Model file for the job. Use its own axes, mm. Face numbers are marked on the shaded views. A direction names the side the tool comes from. Coordinates: 2 decimals unless noted, no trailing zeros. Order: outer loops, then holes, each group sorted by start corner. A loop starts at its lowest first (then second) coordinate and runs counter-clockwise, first axis right, second up.
from build123d import *

# Parameters (mm, degrees)
F1_DEPTH = 31.75
F2_SIZE  = 12
F4_DEPTH = 25.4
F5_R     = 3.175
F6_DEPTH = 25.4
F7_SIZE  = 5.08
F8_R     = 4.200525
F9_DEPTH = 3.175
F10_SIZE = 5.08


with BuildPart() as f1:
    # F0 (on Right) → F1 (new body, symmetric)
    with BuildSketch(Plane.YZ):
        Polygon((-72.2, 15.875), (-72.2, 0), (4, 0), (4, 76.2), (0, 76.2), (0, 6.35), (-66.2, 6.35), (-66.2, 15.875), align=None)
    extrude(amount=F1_DEPTH, both=True)

    # F2
    f2_edges = [f1.edges().sort_by_distance(p)[0] for p in [
        (0, 0, 6.35),
    ]]
    chamfer(f2_edges, length=F2_SIZE)

    # F3 (on Top) → F4 (cut)
    with BuildSketch(Plane.XY):
        with BuildLine():
            Line((-19.05, -21.518925), (-19.05, -72.2))
            Line((-19.05, -72.2), (19.05, -72.2))
            Line((19.05, -72.2), (19.05, -21.518925))
            ThreePointArc((19.05, -21.518925), (0, -8.7), (-19.05, -21.518925))
        make_face()
    extrude(amount=F4_DEPTH, mode=Mode.SUBTRACT)

    # F5 (on face) → F6 (cut)
    with BuildSketch(Plane.XZ):
        with Locations((-15.875, 67.945)):
            Circle(F5_R)
        with Locations((15.875, 67.945)):
            Circle(F5_R)
        with Locations((-15.875, 36.195)):
            Circle(F5_R)
        with Locations((15.875, 36.195)):
            Circle(F5_R)
    extrude(amount=-F6_DEPTH, mode=Mode.SUBTRACT)

    # F7
    f7_edges = [f1.edges().sort_by_distance(p)[0] for p in [
        (-25.4, -66.2, 6.35),
        (25.4, -66.2, 6.35),
    ]]
    chamfer(f7_edges, length=F7_SIZE)

    # F8 (on face) → F9 (cut)
    with BuildSketch(Plane.XZ):
        with Locations((0, 38.1)):
            Circle(F8_R)
    extrude(amount=-F9_DEPTH, mode=Mode.SUBTRACT)

    # F10
    f10_edges = [f1.edges().sort_by_distance(p)[0] for p in [
        (31.75, 2, 76.2),
        (-31.75, 2, 76.2),
        (0, 4, 0),
    ]]
    chamfer(f10_edges, length=F10_SIZE)


solid = f1.part
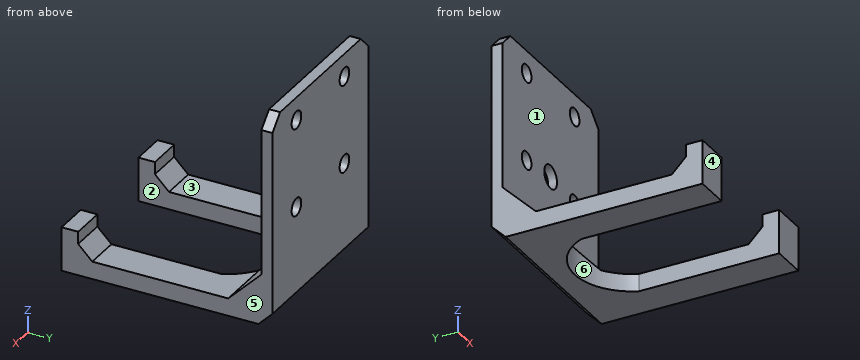
Q1. Mould opens along X. For the marked faces 4, 5 and 6 say: pulls with the +X half, pulls with the -X half, needs draft (parallel to the pull), parting line crosses it, or undercut.
Established:
face 4: needs draft
face 5: pulls with the +X half
face 6: undercut
Q2. Cut at C-C, the plane z = 38.1. List the corners of the cut face in (x, y) (3 decimals), plus the area to 3 significant figures.
Established:
outline: (-31.75, 0) - (-18.415, 0) - (-18.415, 4) - (-31.75, 4) - close; (-13.335, 0) - (-4.201, 0) - (-4.201, 3.175) - (4.201, 3.175) - (4.201, 0) - (13.335, 0) - (13.335, 4) - (-13.335, 4) - close; (18.415, 0) - (31.75, 0) - (31.75, 4) - (18.415, 4) - close
area: 187 mm2
Q3. Which spindle directions (+Z, -Z, +X, -X, +Y, -Y) get a long thin tool onto all of the face, cutting with end or side? Do the marked faces 1, 2 and 3. Say none if no direction does.
Established:
face 1: +Z, +X, -X, -Y
face 2: +Z, -Z, -Y
face 3: +Z, +X, -X
Q4. Cut at A-A, the plane y = -32. List the corners of the cut face in (x, z), plus the area to 3 significant figures.
Established:
outline: (-31.75, 0) - (-19.05, 0) - (-19.05, 6.35) - (-31.75, 6.35) - close; (19.05, 0) - (31.75, 0) - (31.75, 6.35) - (19.05, 6.35) - close
area: 161 mm2
Q5. Cut at D-D, the plane y = -16.5. List the corners of the cut face in (x, z), plus the area to 3 significant figures.
Established:
outline: (-31.75, 0) - (-16.12, 0) - (-16.12, 6.35) - (-31.75, 6.35) - close; (16.12, 0) - (31.75, 0) - (31.75, 6.35) - (16.12, 6.35) - close
area: 198 mm2
Q6. Cut at B-B, the plane x = 0. List the corners of the cut face in (y, z) (3 decimals), plus the area to 3 significant figures.
Established:
outline: (-8.7, 0) - (-1.08, 0) - (4, 5.08) - (4, 76.2) - (0, 76.2) - (0, 42.301) - (3.175, 42.301) - (3.175, 33.899) - (0, 33.899) - (0, 18.35) - (-8.7, 9.65) - close
area: 387 mm2
Q7. Drop flat-ended pins along their axis: P1, Ø3, axis at x = 28, y = -68.5, coming from the +Z side (3 decimals); P2, Ø10.5, axis at x = 24.5, y = -35, coming from the +Z side; P3, Ø4, axis at x = 0, z = 36.5, coming from the -Y side (3 decimals); P4, Ø5.5, axis at x = -15.875, z = 67.945, coming from the -Y side. Give the stop position or say it passes through.
Established:
P1: stops at z = 15.875
P2: stops at z = 6.35
P3: stops at y = 3.175
P4: passes through
Q8. Probe line 1 (Y direction, x = 20.5, z = 38.5); line 2 (Z direction, x = -26.5, y = -15); line 3 (Z direction, x = -19, y = -2.5). List the from-to ranges inside material, lowest first.
Established:
line 1: y = 0 to 4
line 2: z = 0 to 6.35
line 3: z = 0 to 15.85
